Solid Edge part; units mm, degrees
sketch "Sketch1" plane through (0, 0, 0) normal (0, 0, 1) x (1, 0, 0)
  circle A0 centre (0, 0) radius 1.5
  line L0 (-1.4434, 2.5) -> (-2.8868, 0)
  line L1 (-2.8868, 0) -> (-1.4434, -2.5)
  line L2 (-1.4434, -2.5) -> (1.4434, -2.5)
  line L3 (1.4434, -2.5) -> (2.8868, 0)
  line L4 (2.8868, 0) -> (1.4434, 2.5)
  line L5 (1.4434, 2.5) -> (-1.4434, 2.5)
extrude "Protrusion1" add sketch "Sketch1" along normal blind 15
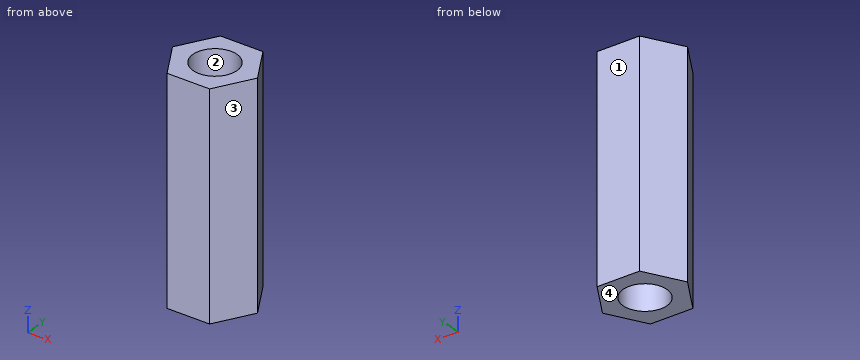
For this review, take the finished solid that the model builds, in its own axes (mm). Face numbers are marked on the shaded views. Coordinates: 2 decimals unless noted, no trailing zeros. Write each loop counter-clockwise with the first axis right and the second up, starting at its lowest first coordinate (ties: lowest second). Pieces come first, ordered by that corner, then holes. Notation, with made-up numbers: (-20.75, -21) - (5.25, -21) arc R7 ccw to (5.25, -12) - close; hole circle Ø1 at (36.5, 54). An arc over 180 degrees is marked (long way). Answer in a Markdown table with one row per item. Add a question column.
Q1. We need section A-A, the plane z = 6.5. State the section outline as (x, y) points.
Q2. For P1, Ø1, axis at x = 2, z = 6, coming from the +Y side; P2, Ø3, axis at y = -2, z = 4, coming from the +X side, all flat-tipped, find the tip position at first contact; note any pin that passes through.
Q3. Draft analysis for pull direction Y (two halves, no side actions). For the marked faces 1, 2, 3 and 4, state which applies: +Y half, -Y half, draft (parallel to the pull), parting line (faces both ways), or undercut.
Q4. For probe 1 along Y at (x, z) = (0, 4.5); probe 2 along Y at (x, z) = (-1.05, 3.5); probe 3 along X at (y, z) = (-1, 4.5), list the stretches that pass through material, from the lowest coordinate up.
Q5. We need section D-D, the plane y = -2.1. State the section outline as (x, z) points.
Q6. We need section C-C, the plane y = -0.35. State the section outline as (x, z) points.
Q7. We need section B-B, the plane x = 0. State the section outline as (y, z) points, and give its area (3 significant figures).
Answer list:
| question | item | result |
|---|---|---|
| 1 | outline | (-2.89, 0) - (-1.44, -2.5) - (1.44, -2.5) - (2.89, 0) - (1.44, 2.5) - (-1.44, 2.5) - close; hole circle Ø3 at (0, 0) |
| 2 | P1 | stops at y = 2.4 |
| 2 | P2 | stops at x = 2.6 |
| 3 | face 1 | +Y half |
| 3 | face 2 | undercut |
| 3 | face 3 | -Y half |
| 3 | face 4 | draft |
| 4 | probe 1 | y = -2.5 to -1.5, 1.5 to 2.5 |
| 4 | probe 2 | y = -2.5 to -1.07, 1.07 to 2.5 |
| 4 | probe 3 | x = -2.31 to -1.12, 1.12 to 2.31 |
| 5 | outline | (-1.67, 0) - (1.67, 0) - (1.67, 15) - (-1.67, 15) - close |
| 6 | outline | (-2.68, 0) - (-1.46, 0) - (-1.46, 15) - (-2.68, 15) - close; (1.46, 0) - (2.68, 0) - (2.68, 15) - (1.46, 15) - close |
| 7 | outline | (-2.5, 0) - (-1.5, 0) - (-1.5, 15) - (-2.5, 15) - close; (1.5, 0) - (2.5, 0) - (2.5, 15) - (1.5, 15) - close |
| 7 | area | 30.0 mm2 |
